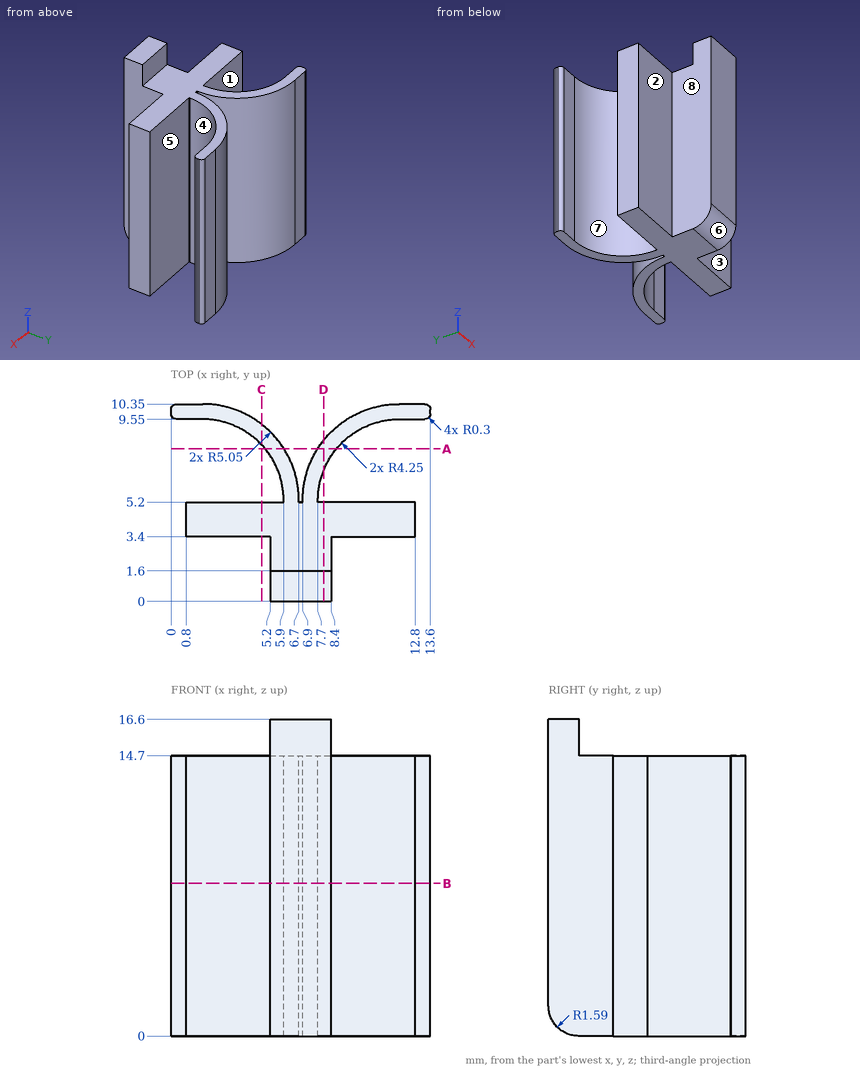
Could you check a few things on this drawing? It's one solid part, dimensions in mm from its lowest x, y, z. A direction names the side the tool comes from. Give positions to 0.01 mm unless a question says otherwise; leave off trailing zeros. Write each loop counter-clockwise with the first axis right and the second up, starting at its lowest first coordinate (ties: lowest second). Pieces come first, ordered by that corner, then holes. Notation, with made-up numbers: (20.25, -38.5) -> (29.25, -38.5) arc R26 ccw to (29.25, -8.5) -> close; hole circle Ø8 at (42.5, 29). An arc over 180 degrees is marked (long way). Write each question's results on one line, items separated by ' | '.
1. I need wall thicknesses on L1, parallel to Y at x = 1, z = 12.5; L2, parallel to X at y = 4.25, z = 9.25; L3, parallel to Z at x = 11.25, y = 4. Which ranges of each line are inside material? Lowest first, please.
Check sheet entries:
L1: y = 3.4 to 5.2, 9.55 to 10.35 | L2: x = 0.8 to 12.8 | L3: z = 0 to 14.7
2. On a 3-axis mill with a long thin cutter (end or side, diameter ignored), from which of +Z, -Z, +X, -X, +Y, -Y can I reach the whole of each face in a straight line? I mean the marked faces 1, 2, 3 and 4. Say none if no direction works.
Check sheet entries:
face 1: +Z, -Z, -X | face 2: +Z, -Z, -X, -Y | face 3: +Z, -Z, +X, -Y | face 4: +Z, -Z, +X
3. If we mould it in two halves opening along Y, with no side actions, what happens to the marked faces 5, 6, 7 and 8? For each: released by +Y, released by -Y, zero draft, split by the parting line, or undercut.
Check sheet entries:
face 5: undercut | face 6: released by -Y | face 7: undercut | face 8: zero draft
4. Will these pins go through, and if not, where does the flat tip stop? pin 1 Ø2 at (x, z) = (2.5, 5.5) entering from -Y; pin 2 Ø2.5 at (y, z) = (2, 12) entering from +X; pin 3 Ø6 at (x, z) = (6.5, 11) entering from +Y.
Check sheet entries:
pin 1: stops at y = 3.4 | pin 2: stops at x = 8.4 | pin 3: stops at y = 10
5. I want a section at A-A, the plane y = 8. Write out the boundary of the cut face in (x, z), then the cut area to 3 significant figures.
Check sheet entries:
outline: (4.93, 0) -> (5.92, 0) -> (5.92, 14.7) -> (4.93, 14.7) -> close; (7.68, 0) -> (8.67, 0) -> (8.67, 14.7) -> (7.68, 14.7) -> close | area: 29.0 mm²
6. I want a section at D-D, the plane x = 8. Write out the boundary of the cut face in (y, z).
Check sheet entries:
outline: (0, 1.59) arc R1.59 ccw to (1.59, 0) -> (5.2, 0) -> (5.2, 14.7) -> (1.6, 14.7) -> (1.6, 16.6) -> (0, 16.6) -> close; (6.87, 0) -> (8.45, 0) -> (8.45, 14.7) -> (6.87, 14.7) -> close
7. I want a section at C-C, the plane x = 4.75. Write out the boundary of the cut face in (y, z), then the cut area to 3 significant figures.
Check sheet entries:
outline: (3.4, 0) -> (5.2, 0) -> (5.2, 14.7) -> (3.4, 14.7) -> close; (8.21, 0) -> (9.29, 0) -> (9.29, 14.7) -> (8.21, 14.7) -> close | area: 42.3 mm²
8. I want a section at B-B, the plane z = 8. Write out the boundary of the cut face in (x, y), then the cut area to 3 significant figures.
Check sheet entries:
outline: (0, 9.85) arc R0.3 ccw to (0.3, 9.55) -> (1.65, 9.55) arc R4.25 cw to (5.9, 5.3) -> (5.9, 5.2) -> (0.8, 5.2) -> (0.8, 3.4) -> (5.2, 3.4) -> (5.2, 0) -> (8.4, 0) -> (8.4, 3.4) -> (12.8, 3.4) -> (12.8, 5.2) -> (7.7, 5.2) -> (7.7, 5.3) arc R4.25 cw to (11.95, 9.55) -> (13.3, 9.55) arc R0.3 ccw to (13.6, 9.85) -> (13.6, 10.05) arc R0.3 ccw to (13.3, 10.35) -> (11.95, 10.35) arc R5.05 ccw to (6.9, 5.3) -> (6.9, 5.2) -> (6.7, 5.2) -> (6.7, 5.3) arc R5.05 ccw to (1.65, 10.35) -> (0.3, 10.35) arc R0.3 ccw to (0, 10.05) -> close | area: 46.9 mm²
